from build123d import *

# Parameters (mm, degrees)
SALIENTE_EXTRUIR1_DEPTH = 3.25
CROQUIS3_W              = 0.48
CROQUIS3_H              = 0.48
SALIENTE_EXTRUIR2_DEPTH = 7
CROQUIS4_W              = 0.48
CROQUIS4_H              = 0.48
SALIENTE_EXTRUIR3_DEPTH = 2
REDONDEO1_R             = 0.5


with BuildPart() as part:
    # Croquis2 → Saliente-Extruir1 (new body)
    with BuildSketch(Plane.XY):
        Polygon((-2.343416672, 0), (2.343416672, 0), (2.343416672, 0.86), (1.34, 1.62), (-1.34, 1.62), (-2.343416672, 0.86), align=None)
    extrude(amount=SALIENTE_EXTRUIR1_DEPTH)

    # Croquis3 → Saliente-Extruir2 (add)
    with BuildSketch(Plane.XY.offset(3.25)):
        with Locations((0, 0.81)):
            Rectangle(CROQUIS3_W, CROQUIS3_H)
        with Locations((1.27, 0.81)):
            Rectangle(CROQUIS3_W, CROQUIS3_H)
        with Locations((-1.27, 0.81)):
            Rectangle(CROQUIS3_W, CROQUIS3_H)
    extrude(amount=SALIENTE_EXTRUIR2_DEPTH)

    # Croquis4 → Saliente-Extruir3 (add)
    with BuildSketch(Plane(origin=(0, 1.05, 0), x_dir=(1, 0, 0), z_dir=(0, 1, 0))):
        with Locations((-1.27, -10.01)):
            Rectangle(CROQUIS4_W, CROQUIS4_H)
        with Locations((0, -10.01)):
            Rectangle(CROQUIS4_W, CROQUIS4_H)
        with Locations((1.27, -10.01)):
            Rectangle(CROQUIS4_W, CROQUIS4_H)
    extrude(amount=SALIENTE_EXTRUIR3_DEPTH)

    # Redondeo1
    redondeo1_edges = [part.edges().sort_by_distance(p)[0] for p in [
        (0, 0.57, 10.25),
        (1.27, 0.57, 10.25),
        (-1.27, 0.57, 10.25),
    ]]
    fillet(redondeo1_edges, radius=REDONDEO1_R)


solid = part.part
Model file for the job. Use its own axes, mm. A direction names the side the tool comes from. Give positions to 0.01 mm unless a question says otherwise; leave off trailing zeros. Write each loop counter-clockwise with the first axis right and the second up, starting at its lowest first coordinate (ties: lowest second). Pieces come first, ordered by that corner, then holes. Notation, with made-up numbers: M 0.5,-7.75 L 58.5,-7.75 A20 ccw 58.5,21.25 Z; hole C -17.75,74 d10. An arc over 180 degrees is marked long. One line per item, written item: value. Start each with the question number.
Q1. Two-plate mould, pull along X, no slides. Class faces 5 (the flat face through (0, 1, 0)), 6 (the flat face through (1.03, 0.9, 7.3)), 7 (the flat face through (1.51, 0.9, 7.3)): +X half, -X half, draft (parallel to the pull), parting line (faces both ways), or undercut.
Q2. Probe probe 1 along Z at (x, y) = (-1.1, 1.4); probe 2 along X at (y, z) = (0.6, 4.25); probe 3 along Z at (x, y) = (-0.65, 1.1). List the from-to ranges inside material, lowest first. Write a range as [from, to].
Q3. 3-axis set-ups, long thin cutter, end or side, ignore diameter. For faces 1 (the flat face through (-1.51, 0.8, 7.5)), 2 (the flat face through (-0.24, 0.9, 7.3)), 3 (the flat face through (-1.83, 1.25, 1.6)), 4 (the flat face through (0, 1.62, 2)): which of +Z, -Z, +X, -X, +Y, -Y reach the whole face in a straight line?
Q4. Saw through at B-B, the plane z = 3.5. Write the cut outline in (x, y), plus the area to 3 significant figures.
Q5. Saw through at A-A, the plane y = 2.75. Write the cut outline in (x, z).
Q6. Saw through at C-C, the plane z = 1.5. Write the cut outline in (x, y).
Q7. Saw through at D-D, the plane y = 1.5. Write the cut outline in (x, z), plus the area to 3 significant figures.
Q8. Drop flat-ended pins along their axis: pin 1 Ø1.5 at (y, z) = (0.5, 4.5) entering from +X; pin 2 Ø0.5 at (x, y) = (1.5, 2) entering from -Z; pin 3 Ø0.5 at (x, z) = (-1, 7) entering from +Y. Give the stop position or say it passes through.
Output values:
1. face 5: draft
1. face 6: undercut
1. face 7: +X half
2. probe 1: z = [0, 3.25], [9.77, 10.25]
2. probe 2: x = [-1.51, -1.03], [-0.24, 0.24], [1.03, 1.51]
2. probe 3: z = [0, 3.25]
3. face 1: +Z, -X, +Y, -Y
3. face 2: +Z, +Y, -Y
3. face 3: -Z, -X, +Y
3. face 4: -Z, +X, -X, +Y
4. outline: M -1.51,0.57 L -1.03,0.57 L -1.03,1.05 L -1.51,1.05 Z; M -0.24,0.57 L 0.24,0.57 L 0.24,1.05 L -0.24,1.05 Z; M 1.03,0.57 L 1.51,0.57 L 1.51,1.05 L 1.03,1.05 Z
4. area: 0.691 mm²
5. outline: M -1.51,9.77 L -1.03,9.77 L -1.03,10.25 L -1.51,10.25 Z; M -0.24,9.77 L 0.24,9.77 L 0.24,10.25 L -0.24,10.25 Z; M 1.03,9.77 L 1.51,9.77 L 1.51,10.25 L 1.03,10.25 Z
6. outline: M -2.34,0 L 2.34,0 L 2.34,0.86 L 1.34,1.62 L -1.34,1.62 L -2.34,0.86 Z
7. outline: M -1.51,9.77 L -1.03,9.77 L -1.03,10.25 L -1.51,10.25 Z; M -1.5,0 L 1.5,0 L 1.5,3.25 L -1.5,3.25 Z; M -0.24,9.77 L 0.24,9.77 L 0.24,10.25 L -0.24,10.25 Z; M 1.03,9.77 L 1.51,9.77 L 1.51,10.25 L 1.03,10.25 Z
7. area: 10.4 mm²
8. pin 1: stops at x = 1.51
8. pin 2: stops at z = 9.77
8. pin 3: stops at y = 1.05
